CAD build for the part. Positions are in the model's coordinates, mm. A direction names the side the tool comes from. Give positions to 0.01 mm unless a question says otherwise; leave off trailing zeros. Write each loop counter-clockwise with the first axis right and the second up, starting at its lowest first coordinate (ties: lowest second). Pieces come first, ordered by that corner, then holes. Notation, with made-up numbers: (81.5, 82) - (128.5, 82) arc R27 cw to (128.5, 106) - close; hole circle Ø10 at (75, 79.5). An arc over 180 degrees is marked (long way). Answer as a JSON object with one key per item and string values.
from build123d import *

# Parameters (mm, degrees)
SKETCH1_R           = 3.96875
BOSS_EXTRUDE1_DEPTH = 3.175
FILLET1_R           = 12.7


with BuildPart() as part:
    # Sketch1 → Boss-Extrude1 (new body)
    with BuildSketch(Plane.XY):
        Polygon((0, 0), (-120.65, 81.227610635), (-120.65, 29.17348858), (0, -52.054122056), (120.65, 29.17348858), (120.65, 81.227610635), align=None)
        with Locations((-95.25, 38.1)):
            Circle(SKETCH1_R, mode=Mode.SUBTRACT)
        with Locations((95.25, 38.1)):
            Circle(SKETCH1_R, mode=Mode.SUBTRACT)
        with Locations((-12.7, -17.476786224)):
            Circle(SKETCH1_R, mode=Mode.SUBTRACT)
        with Locations((12.7, -17.476786224)):
            Circle(SKETCH1_R, mode=Mode.SUBTRACT)
    extrude(amount=BOSS_EXTRUDE1_DEPTH)

    # Fillet1
    fillet1_edges = [part.edges().sort_by_distance(p)[0] for p in [
        (120.65, 81.227610635, 1.5875),
        (120.65, 29.17348858, 1.5875),
        (0, -52.054122056, 1.5875),
        (-120.65, 29.17348858, 1.5875),
        (-120.65, 81.227610635, 1.5875),
        (0, 0, 1.5875),
    ]]
    fillet(fillet1_edges, radius=FILLET1_R)


solid = part.part
(1) Probe L1, parallel to X at y = -16, z = 0.5; L2, parallel to X at y = 6, z = 3.05; L3, parallel to Y at x = 98, z = 0.6. List the from-to ranges inside material, lowest first. Write a range as [from, to].
Answer key:
{"L1": "x = [-53.55, -16.38], [-9.02, 9.02], [16.38, 53.55]", "L2": "x = [-86.23, -8.91], [8.91, 86.23]", "L3": "y = [13.92, 35.24], [40.96, 65.98]"}
(2) Saw through at D-D, the plane y = 38.1. Give the cut face in (x, z) (3 decimals).
Answer key:
{"outline": "(-120.65, 0) - (-99.219, 0) - (-99.219, 3.175) - (-120.65, 3.175) - close; (-91.281, 0) - (-56.591, 0) - (-56.591, 3.175) - (-91.281, 3.175) - close; (56.591, 0) - (91.281, 0) - (91.281, 3.175) - (56.591, 3.175) - close; (99.219, 0) - (120.65, 0) - (120.65, 3.175) - (99.219, 3.175) - close"}
(3) Saw through at C-C, the plane x = -12.7. Give the cut face in (y, z) (3 decimals), and give its area (3 significant figures).
Answer key:
{"outline": "(-43.504, 0) - (-21.446, 0) - (-21.446, 3.175) - (-43.504, 3.175) - close; (-13.508, 0) - (8.55, 0) - (8.55, 3.175) - (-13.508, 3.175) - close", "area": "140 mm²"}
(4) 3-axis set-ups, long thin cutter, end or side, ignore diameter. For faces 1 (the face through (54.63, 36.78, 1.57)), 2 (the face through (-10.87, -21, 1.57)): which of +Z, -Z, +X, -X, +Y, -Y reach the whole face in a straight line?
Answer key:
{"face 1": "+Z, -Z, +Y", "face 2": "+Z, -Z"}
(5) Saw through at B-B, the plane z = 2.55. Give the cut face in (x, y), and give its area (3 significant figures).
Answer key:
{"outline": "(-120.65, 35.93) arc R12.7 ccw to (-115.04, 25.4) - (-7.09, -47.28) arc R12.7 ccw to (7.09, -47.28) - (115.04, 25.4) arc R12.7 ccw to (120.65, 35.93) - (120.65, 57.37) arc R12.7 ccw to (100.86, 67.9) - (7.09, 4.78) arc R12.7 cw to (-7.09, 4.78) - (-100.86, 67.9) arc R12.7 ccw to (-120.65, 57.37) - close; hole circle Ø7.94 at (-95.25, 38.1); hole circle Ø7.94 at (-12.7, -17.48); hole circle Ø7.94 at (12.7, -17.48); hole circle Ø7.94 at (95.25, 38.1)", "area": "12,100 mm²"}
(6) Pull direction X, two halves, no side cores. Call faces 3 (the face through (119.2, 30.04, 1.61)), 4 (the face through (-2, -2, 0)), 5 (the face through (-53.32, 35.9, 1.57)): pulls with the +X half, pulls with the -X half, needs draft (parallel to the pull), parting line crosses it, or undercut.
Answer key:
{"face 3": "pulls with the +X half", "face 4": "needs draft", "face 5": "undercut"}
(7) Saw through at A-A, the plane y = 15. Give the cut face in (x, z) (3 decimals).
Answer key:
{"outline": "(-99.598, 0) - (-22.28, 0) - (-22.28, 3.175) - (-99.598, 3.175) - close; (22.28, 0) - (99.598, 0) - (99.598, 3.175) - (22.28, 3.175) - close"}
